Design review of the part built by this model. Coordinates are the model's own, in mm. A direction names the side the tool comes from. Give positions to 0.01 mm unless a question says otherwise; leave off trailing zeros. Write each loop counter-clockwise with the first axis right and the second up, starting at its lowest first coordinate (ties: lowest second). Pieces come first, ordered by that corner, then holes.
```python
from build123d import *

# Parameters (mm, degrees)
SKETCH1_R           = 4
SKETCH1_R_2         = 2
BOSS_EXTRUDE1_DEPTH = 6
FILLET2_R           = 5
FILLET3_R           = 3.9


with BuildPart() as part:
    # Sketch1 → Boss-Extrude1 (new body)
    with BuildSketch(Plane(origin=(0, 0, 0), x_dir=(1, 0, 0), z_dir=(0, 1, 0))):
        Polygon((-23, 0), (23, 0), (23, 19), (15, 19), (15, 50), (-15, 50), (-15, 19), (-23, 19), align=None)
        with Locations(Location((0, 40, 0), (0, 0, 270))):
            Circle(SKETCH1_R, mode=Mode.SUBTRACT)
        with Locations(Location((11, 9, 0), (0, 0, 270))):
            Circle(SKETCH1_R_2, mode=Mode.SUBTRACT)
        with Locations(Location((-11, 9, 0), (0, 0, 90))):
            Circle(SKETCH1_R_2, mode=Mode.SUBTRACT)
    extrude(amount=BOSS_EXTRUDE1_DEPTH)

    # Fillet2
    fillet2_edges = [part.edges().sort_by_distance(p)[0] for p in [
        (15, 3, -50),
        (23, 3, 0),
        (-23, 3, 0),
        (-15, 3, -50),
    ]]
    fillet(fillet2_edges, radius=FILLET2_R)

    # Fillet3
    fillet3_edges = [part.edges().sort_by_distance(p)[0] for p in [
        (15, 3, -19),
        (23, 3, -19),
        (-23, 3, -19),
        (-15, 3, -19),
    ]]
    fillet(fillet3_edges, radius=FILLET3_R)


solid = part.part
```
(1) Consider section A-A, the plane x = 0. Give the boundary of the cut face in (y, z), then the cut area to 3 significant figures.
Resolved:
outline: (0, -50) - (6, -50) - (6, -44) - (0, -44) - close; (0, -36) - (6, -36) - (6, 0) - (0, 0) - close
area: 252 mm2
(2) Clearance check with flat-ended pins moving along their axes: P1, Ø3, axis at x = 17, z = -28, coming from the +Y side; P2, Ø1.8, axis at y = 1.5, z = -29, coming from the +X side. State where each tip first meets the part, or that it passes through.
Resolved:
P1: passes through
P2: stops at x = 15
(3) Consider section B-B, the plane z = -9. Give the boundary of the cut face in (x, y).
Resolved:
outline: (-23, 0) - (-13, 0) - (-13, 6) - (-23, 6) - close; (-9, 0) - (9, 0) - (9, 6) - (-9, 6) - close; (13, 0) - (23, 0) - (23, 6) - (13, 6) - close
(4) Mouldability with a two-part tool opening along Z and no side actions: class faces 4 (the face through (-12.352, 2.958, -7.526)), 5 (the face through (-14, 3, -48)), 6 (the face through (21, 3, -1)) as pulls with the +Z half, pulls with the -Z half, needs draft (parallel to the pull), parting line crosses it, or undercut.
Resolved:
face 4: undercut
face 5: pulls with the -Z half
face 6: pulls with the +Z half
(5) Tool access review of faces 1 (the face through (-15, 3, -34)), 2 (the face through (-23, 3, -10)), 3 (the face through (15, 3, -34)): name each direction out of +Z, -Z, +X, -X, +Y, -Y from which nothing blocks a thin tool from reaching the whole face with its end or side.
Resolved:
face 1: -Z, -X, +Y, -Y
face 2: +Z, -Z, -X, +Y, -Y
face 3: -Z, +X, +Y, -Y
(6) To check wall thickness, follow L1, parallel to X at y = 4.45, z = -9; L2, parallel to X at y = 3.65, z = -35.5; L3, parallel to Z at x = -12, y = 1.3. State the ranges of each line that lie inside material, in increasing order.
Resolved:
L1: x = -23 to -13, -9 to 9, 13 to 23
L2: x = -15 to 15
L3: z = -49.58 to -10.73, -7.27 to 0
(7) Consider section D-D, the plane z = -40. Give the boundary of the cut face in (x, y), then the cut area to 3 significant figures.
Resolved:
outline: (-15, 0) - (-4, 0) - (-4, 6) - (-15, 6) - close; (4, 0) - (15, 0) - (15, 6) - (4, 6) - close
area: 132 mm2
(8) Consider section C-C, the plane y = 0.9. Give the boundary of the cut face in (x, z).
Resolved:
outline: (-23, -15.1) arc R3.9 ccw to (-19.1, -19) - (-18.9, -19) arc R3.9 cw to (-15, -22.9) - (-15, -45) arc R5 ccw to (-10, -50) - (10, -50) arc R5 ccw to (15, -45) - (15, -22.9) arc R3.9 cw to (18.9, -19) - (19.1, -19) arc R3.9 ccw to (23, -15.1) - (23, -5) arc R5 ccw to (18, 0) - (-18, 0) arc R5 ccw to (-23, -5) - close; hole circle Ø4 at (-11, -9); hole circle Ø8 at (0, -40); hole circle Ø4 at (11, -9)
